Build history of the part. All positions in model axes, mm. Face numbers are marked on the shaded views. A direction names the side the tool comes from. Round coordinates to 2 decimals unless told otherwise and drop trailing zeros. Order: outer loops, then holes, each group sorted by start corner. A loop starts at its lowest first (then second) coordinate and runs counter-clockwise, first axis right, second up. Notation, with made-up numbers: (80.5, -32.5) - (136.5, -32.5) arc R11 cw to (136.5, -20.5) - close; hole circle Ø10 at (53, -6.75). An arc over 180 degrees is marked (long way). One line per question, with ' | ' between items. Start each with the question number.
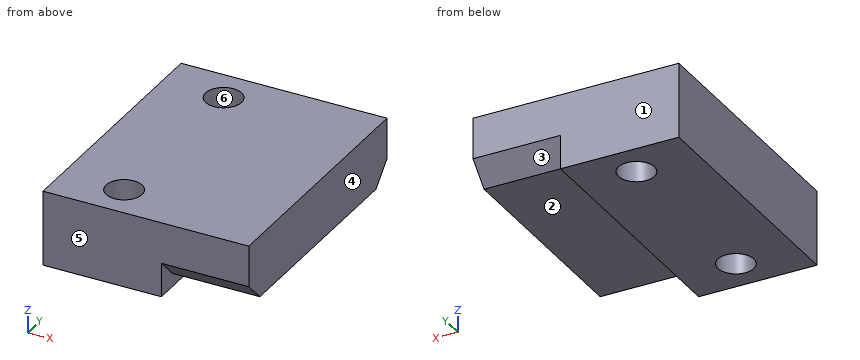
from build123d import *

# Parameters (mm, degrees)
BOSS_EXTRUDE1_DEPTH = 12.5
SKETCH2_R           = 1.75
CUT_EXTRUDE1_DEPTH  = 18.59374889
CHAMFER1_SIZE       = 2


with BuildPart() as part:
    # Sketch1 → Boss-Extrude1 (new, symmetric)
    with BuildSketch(Plane(origin=(0, 0, 0), x_dir=(1, 0, 0), z_dir=(0, 1, 0))):
        Polygon((-10, 7.3), (1.5, 7.3), (1.5, 6), (10, 6), (10, 0), (-10, 0), align=None)
    extrude(amount=BOSS_EXTRUDE1_DEPTH, both=True)

    # Sketch2 → Cut-Extrude1 (cut, through all)
    with BuildSketch(Plane.XY):
        with Locations((-4, 9)):
            Circle(SKETCH2_R)
        with Locations((-4, -9)):
            Circle(SKETCH2_R)
    extrude(amount=-CUT_EXTRUDE1_DEPTH, mode=Mode.SUBTRACT)

    # Chamfer1
    chamfer1_edges = [part.edges().sort_by_distance(p)[0] for p in [
        (5.75, 12.5, -6),
        (5.75, -12.5, -6),
    ]]
    chamfer(chamfer1_edges, length=CHAMFER1_SIZE)


solid = part.part
Item 1: Slice it at A-A (x = -4). Write the cut outline in (y, z), plus the area to 3 significant figures.
Item 2: Slice it at B-B (y = -9). Write the cut outline in (x, z), plus the area to 3 significant figures.
Item 3: Pull direction Y, two halves, no side cores. Call the marked faces 3, 4, 5 and 6: released by +Y, released by -Y, zero draft, split by the parting line, or undercut.
Item 4: Slice it at C-C (z = -4.5). Write the cut outline in (x, y), plus the area to 3 significant figures.
Item 5: 3-axis set-ups, long thin cutter, end or side, ignore diameter. For the marked faces 1 and 2: which of +Z, -Z, +X, -X, +Y, -Y reach the whole face in a straight line?
Item 6: Slice it at D-D (y = 6.25). Write the cut outline in (x, z).
Item 7: Pin check, flat tips, straight feed: pin 1 (2 mm diameter, centred on x = -4, y = 9, fed in from +Z); pin 2 (2.5 mm diameter, centred on x = 5, y = -3, fed in from -Z). Stop position of each tip, or through.
Item 8: Wall check: line 1 along Y through (x, z) = (-4, -3.5); line 2 along Z through (x, y) = (4.25, 10.75); line 3 along Z through (x, y) = (2, 3.5). Give the ranges that are in metal, low to high. Write a range as [from, to].
A:
1) outline: (-12.5, -7.3) - (-10.75, -7.3) - (-10.75, 0) - (-12.5, 0) - close; (-7.25, -7.3) - (7.25, -7.3) - (7.25, 0) - (-7.25, 0) - close; (10.75, -7.3) - (12.5, -7.3) - (12.5, 0) - (10.75, 0) - close | area: 131 mm^2
2) outline: (-10, -7.3) - (-5.75, -7.3) - (-5.75, 0) - (-10, 0) - close; (-2.25, -7.3) - (1.5, -7.3) - (1.5, -6) - (10, -6) - (10, 0) - (-2.25, 0) - close | area: 109 mm^2
3) face 3: released by +Y | face 4: zero draft | face 5: released by -Y | face 6: undercut
4) outline: (-10, -12.5) - (1.5, -12.5) - (1.5, -12) - (10, -12) - (10, 12) - (1.5, 12) - (1.5, 12.5) - (-10, 12.5) - close; hole circle Ø3.5 at (-4, -9); hole circle Ø3.5 at (-4, 9) | area: 472 mm^2
5) face 1: +Z, -Z, +X, -X, +Y | face 2: -Z, +X, +Y, -Y
6) outline: (-10, -7.3) - (1.5, -7.3) - (1.5, -6) - (10, -6) - (10, 0) - (-10, 0) - close
7) pin 1: through | pin 2: z = -6
8) line 1: [-12.5, -10.75], [-7.25, 7.25], [10.75, 12.5] | line 2: [-5.75, 0] | line 3: [-6, 0]
